```python
from build123d import *

# Parameters (mm, degrees)
F1_DEPTH = 22.86
F2_R     = 5.08
F3_R     = 3.175
F4_DEPTH = 2.54
F5_R     = 3.175
F6_DEPTH = 2.54


with BuildPart() as f1:
    # F0 (on Front) → F1 (new body, symmetric)
    with BuildSketch(Plane.XZ):
        with BuildLine():
            Line((20.637052, 16.137419), (-12.382948, 16.137419))
            ThreePointArc((-12.382948, 16.137419), (-16.873076, 14.277547), (-18.732948, 9.787419))
            Line((-18.732948, 9.787419), (-18.732948, -23.232581))
            ThreePointArc((-18.732948, -23.232581), (-16.873076, -27.722709), (-12.382948, -29.582581))
            Line((-12.382948, -29.582581), (20.637052, -29.582581))
            ThreePointArc((20.637052, -29.582581), (25.12718, -27.722709), (26.987052, -23.232581))
            Line((26.987052, -23.232581), (26.987052, 9.787419))
            ThreePointArc((26.987052, 9.787419), (25.12718, 14.277547), (20.637052, 16.137419))
        make_face()
    extrude(amount=F1_DEPTH, both=True)

    # F2
    f2_edges = [f1.edges().sort_by_distance(p)[0] for p in [
        (4.127052, -22.86, 16.137419),
        (4.127052, 22.86, 16.137419),
    ]]
    fillet(f2_edges, radius=F2_R)

    # F3 (on face) → F4 (cut)
    with BuildSketch(Plane(origin=(-18.732948, 0, 0), x_dir=(0, -1, 0), z_dir=(-1, 0, 0))):
        with Locations((0, -6.722581)):
            Circle(F3_R)
    extrude(amount=-F4_DEPTH, mode=Mode.SUBTRACT)

    # F5 (on face) → F6 (cut)
    with BuildSketch(Plane.YZ.offset(26.987052)):
        with Locations((-7.62, 2.167419)):
            Circle(F5_R)
        with Locations((7.62, 2.167419)):
            Circle(F5_R)
        with Locations((7.62, -6.722581)):
            Circle(F5_R)
        with Locations((-7.62, -6.722581)):
            Circle(F5_R)
        with Locations((-7.62, -15.612581)):
            Circle(F5_R)
        with Locations((7.62, -15.612581)):
            Circle(F5_R)
    extrude(amount=-F6_DEPTH, mode=Mode.SUBTRACT)


solid = f1.part
```
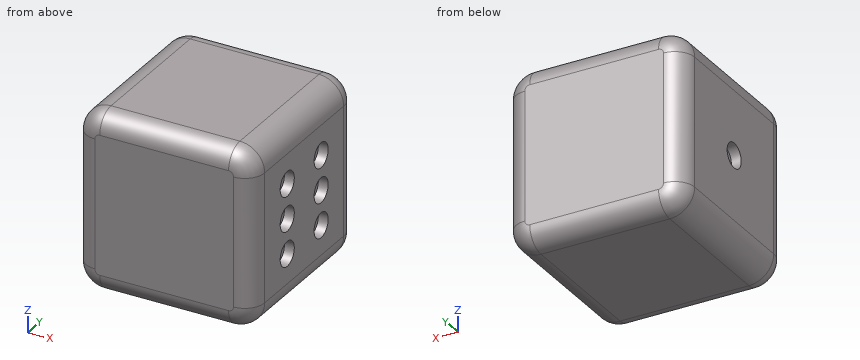
Here's how the part is built. I have some questions about the finished solid (model axes, mm). Round coordinates to 2 decimals unless told otherwise and drop trailing zeros. Order: outer loops, then holes, each group sorted by start corner. A loop starts at its lowest first (then second) coordinate and runs counter-clockwise, first axis right, second up. Notation, with made-up numbers: M 18.25,74 L 71.25,74 A19 ccw 71.25,79 Z; hole C 76.25,42 d9. An arc over 180 degrees is marked long. One line per question, with ' | ' between items.
1) I want a section at D-D, the plane z = 1.5. Write out the boundary of the cut face in (x, y), then the cut area to 3 significant figures.
Working result:
outline: M -18.73,-17.78 A5.08 ccw -13.65,-22.86 L 21.91,-22.86 A5.08 ccw 26.99,-17.78 L 26.99,-10.72 L 24.45,-10.72 L 24.45,-4.52 L 26.99,-4.52 L 26.99,4.52 L 24.45,4.52 L 24.45,10.72 L 26.99,10.72 L 26.99,17.78 A5.08 ccw 21.91,22.86 L -13.65,22.86 A5.08 ccw -18.73,17.78 Z | area: 2,040 mm²
2) For pin 1 Ø4 at (y, z) = (7.62, -15.61) entering from +X, with a flat end and sliding along its axis, tell me the tip position at first contact or that it passes through.
Working result:
pin 1: x = 24.45
3) I want a section at C-C, the plane y = -14. Write out the boundary of the cut face in (x, z).
Working result:
outline: M -18.73,-23.23 A6.35 ccw -12.38,-29.58 L 20.64,-29.58 A6.35 ccw 26.99,-23.23 L 26.99,9.79 A6.35 ccw 20.64,16.14 L -12.38,16.14 A6.35 ccw -18.73,9.79 Z
4) I need wall thicknesses on line 1 along Z through (x, y) = (25.2, -7.62); line 2 along Z through (x, y) = (25, 7); line 3 along Z through (x, y) = (21, 17). Which ranges of each line are inside material? Lowest first, please.
Working result:
line 1: -27.65 to -18.79, -12.44 to -9.9, -3.55 to -1.01, 5.34 to 14.2 | line 2: -27.85 to -18.73, -12.5 to -9.84, -3.61 to -0.95, 5.28 to 14.4 | line 3: -29.57 to 16.13
5) I want a section at B-B, the plane z = -8. Write out the boundary of the cut face in (x, y).
Working result:
outline: M -18.73,-17.78 A5.08 ccw -13.65,-22.86 L 21.91,-22.86 A5.08 ccw 26.99,-17.78 L 26.99,-10.53 L 24.45,-10.53 L 24.45,-4.71 L 26.99,-4.71 L 26.99,4.71 L 24.45,4.71 L 24.45,10.53 L 26.99,10.53 L 26.99,17.78 A5.08 ccw 21.91,22.86 L -13.65,22.86 A5.08 ccw -18.73,17.78 L -18.73,2.91 L -16.19,2.91 L -16.19,-2.91 L -18.73,-2.91 Z
6) I want a section at A-A, the plane y = -7.62. Write out the boundary of the cut face in (x, z).
Working result:
outline: M -18.73,-23.23 A6.35 ccw -12.38,-29.58 L 20.64,-29.58 A6.35 ccw 26.99,-23.23 L 26.99,-18.79 L 24.45,-18.79 L 24.45,-12.44 L 26.99,-12.44 L 26.99,-9.9 L 24.45,-9.9 L 24.45,-3.55 L 26.99,-3.55 L 26.99,-1.01 L 24.45,-1.01 L 24.45,5.34 L 26.99,5.34 L 26.99,9.79 A6.35 ccw 20.64,16.14 L -12.38,16.14 A6.35 ccw -18.73,9.79 Z
